Model file for the job. Use its own axes, mm. Round coordinates to 2 decimals unless told otherwise and drop trailing zeros. Order: outer loops, then holes, each group sorted by start corner. A loop starts at its lowest first (then second) coordinate and runs counter-clockwise, first axis right, second up. Notation, with made-up numbers: (-25, 35.25) - (27, 35.25) arc R18 cw to (27, 68.25) - close; hole circle Ø11 at (-10.5, 82.5). An arc over 180 degrees is marked (long way). Use one line per item in the form item = value.
Autodesk Inventor part; units mm, degrees
ref_plane "作業平面1" through (0, -9, 0) normal (0, 1, 0) x (-1, 0, 0)
ref_plane "YZ Plane" through (0, 0, 0) normal (1, 0, 0) x (0, 1, 0)
ref_plane "XY Plane" through (0, 0, 0) normal (0, 0, 1) x (1, 0, 0)
sketch "スケッチ1" plane through (0, 0, 0) normal (1, 0, 0) x (0, 1, 0)
  circle A0 centre (0, 0) radius 9
  circle A1 centre (0, 0) radius 6.5
  dimension "d0" = 18
  dimension "d1" = 13
extrude "押し出し1" add sketch "スケッチ1" along normal blind 280
ref_plane "作業平面1" through (0, -9, 0) normal (0, 1, 0) x (-1, 0, 0)
sketch "スケッチ2" plane through (0, -9, 0) normal (0, 1, 0) x (-1, 0, 0)
  line L0 (0, 9) -> (0, -9)
  line L1 (-280, 9) -> (-280, -9)
  point P0 (0, 0)
  point P1 (-7.5, 0)
  point P2 (-272.5, 0)
  dimension "d4" = 7.5
  dimension "d5" = 7.5
hole "穴1" at (7.5, -9, 0) at (272.5, -9, 0) direction (0, 1, 0) diameter 3.4 end through all
properties part number "roller-hand-v1-roller" material "PVC 配管"
(1) Slice it at A-A on y = 2. Give the cut face in (x, z), then the cut area to 3 significant figures.
Report:
outline = (0, -8.77) - (280, -8.77) - (280, -6.18) - (0, -6.18) - close; (0, 6.18) - (280, 6.18) - (280, 8.77) - (0, 8.77) - close
area = 1,450 mm2
(2) Slice it at B-B on x = 29. Give the cut face in (y, z).
Report:
outline = circle Ø18 at (0, 0); hole circle Ø13 at (0, 0)
(3) Pin check, flat tips, straight feed: pin 1 (1 mm diameter, centred on x = 123.5, y = 3, fed in from -Z); pin 2 (2 mm diameter, centred on x = 175, z = 3.5, fed in from +Y); pin 3 (1.5 mm diameter, centred on x = 98, z = 3.5, fed in from -Y). Stop position of each tip, or through.
Report:
pin_1 = -8.65
pin_2 = 8.65
pin_3 = -8.57
(4) Pull direction Z, two halves, no side cores. Call faces 1 (the face through (0, 3, -6)), 2 (the face through (138.04, -1.172, -8.923)), 3 (the face through (138.04, -5.158, 3.955)): released by +Z, released by -Z, zero draft, split by the parting line, or undercut.
Report:
face_1 = zero draft
face_2 = split by the parting line
face_3 = undercut
(5) Probe probe 1 along X at (y, z) = (7.6, 0); probe 2 along Y at (x, z) = (19.5, 0.25); probe 3 along Z at (x, y) = (57.5, -0.5). List the from-to ranges inside material, lowest first. Write a range as [from, to].
Report:
probe_1 = [0, 5.8], [9.2, 270.8], [274.2, 280]
probe_2 = [-9, -6.5], [6.5, 9]
probe_3 = [-8.99, -6.48], [6.48, 8.99]
